Could you check a few things on this model? Use its own coordinates, in mm. Face numbers are marked on the shaded views. Round coordinates to 2 decimals unless told otherwise and drop trailing zeros. Loops run counter-clockwise (first coordinate to the right, second up) from the corner with the lowest first, then second, coordinate; pieces in that order, holes last. Notation, with made-up numbers: (84, 59.25) -> (92, 59.25) arc R36 ccw to (92, 95.25) -> close; hole circle Ø5 at (20, -17.5). An arc over 180 degrees is marked (long way). Write each question's results on one line, items separated by ' | '.
from build123d import *

# Parameters (mm, degrees)
SKETCH1_W           = 37.9349
SKETCH1_H           = 37.9349
BOSS_EXTRUDE1_DEPTH = 3.175
SKETCH9_R           = 1.1176
SKETCH9_R_2         = 6.35
CUT_EXTRUDE2_DEPTH  = 3.175


with BuildPart() as part:
    # Sketch1 → Boss-Extrude1 (new body)
    with BuildSketch(Plane.XY):
        with Locations((18.96745, 18.96745)):
            Rectangle(SKETCH1_W, SKETCH1_H)
    extrude(amount=BOSS_EXTRUDE1_DEPTH)

    # Sketch9 → Cut-Extrude2 (cut)
    with BuildSketch(Plane.XY.offset(3.175)):
        with Locations((33.62325, 33.62325)):
            Circle(SKETCH9_R)
        with Locations((4.31165, 33.62325)):
            Circle(SKETCH9_R)
        with Locations((4.31165, 4.31165)):
            Circle(SKETCH9_R)
        with Locations((33.62325, 4.31165)):
            Circle(SKETCH9_R)
        with Locations((18.96745, 18.96745)):
            Circle(SKETCH9_R_2)
        with BuildLine():
            Line((35.385619933, 12.100169933), (35.385619933, 2.549280067))
            Line((35.385619933, 2.549280067), (25.834730067, 2.549280067))
            ThreePointArc((25.834730067, 2.549280067), (25.2984, 2.01295), (25.834730067, 1.476619933))
            Line((25.834730067, 1.476619933), (35.385619933, 1.476619933))
            ThreePointArc((35.385619933, 1.476619933), (37.303202335, 0.631697665), (36.458280067, 2.549280067))
            Line((36.458280067, 2.549280067), (36.458280067, 12.100169933))
            ThreePointArc((36.458280067, 12.100169933), (35.92195, 12.6365), (35.385619933, 12.100169933))
        make_face()
        with BuildLine():
            Line((35.385619933, 36.458280067), (25.834730067, 36.458280067))
            ThreePointArc((25.834730067, 36.458280067), (25.2984, 35.92195), (25.834730067, 35.385619933))
            Line((25.834730067, 35.385619933), (35.385619933, 35.385619933))
            Line((35.385619933, 35.385619933), (35.385619933, 25.834730067))
            ThreePointArc((35.385619933, 25.834730067), (35.92195, 25.2984), (36.458280067, 25.834730067))
            Line((36.458280067, 25.834730067), (36.458280067, 35.385619933))
            ThreePointArc((36.458280067, 35.385619933), (37.303202335, 37.303202335), (35.385619933, 36.458280067))
        make_face()
        with BuildLine():
            Line((12.048880067, 36.458280067), (2.549280067, 36.458280067))
            ThreePointArc((2.549280067, 36.458280067), (0.631697665, 37.303202335), (1.476619933, 35.385619933))
            Line((1.476619933, 35.385619933), (1.476619933, 25.886019933))
            ThreePointArc((1.476619933, 25.886019933), (2.01295, 25.349689867), (2.549280067, 25.886019933))
            Line((2.549280067, 25.886019933), (2.549280067, 35.385619933))
            Line((2.549280067, 35.385619933), (12.048880067, 35.385619933))
            ThreePointArc((12.048880067, 35.385619933), (12.585210133, 35.92195), (12.048880067, 36.458280067))
        make_face()
        with BuildLine():
            Line((23.06955, 36.458280067), (14.86535, 36.458280067))
            ThreePointArc((14.86535, 36.458280067), (14.329019933, 35.92195), (14.86535, 35.385619933))
            Line((14.86535, 35.385619933), (23.06955, 35.385619933))
            ThreePointArc((23.06955, 35.385619933), (23.605880067, 35.92195), (23.06955, 36.458280067))
        make_face()
        with BuildLine():
            Line((2.549280067, 23.06955), (2.549280067, 14.86535))
            ThreePointArc((2.549280067, 14.86535), (2.01295, 14.329019933), (1.476619933, 14.86535))
            Line((1.476619933, 14.86535), (1.476619933, 23.06955))
            ThreePointArc((1.476619933, 23.06955), (2.01295, 23.605880067), (2.549280067, 23.06955))
        make_face()
        with BuildLine():
            Line((36.458280067, 23.06955), (36.458280067, 14.86535))
            ThreePointArc((36.458280067, 14.86535), (35.92195, 14.329019933), (35.385619933, 14.86535))
            Line((35.385619933, 14.86535), (35.385619933, 23.06955))
            ThreePointArc((35.385619933, 23.06955), (35.92195, 23.605880067), (36.458280067, 23.06955))
        make_face()
        with BuildLine():
            Line((23.06955, 2.549280067), (14.86535, 2.549280067))
            ThreePointArc((14.86535, 2.549280067), (14.329019933, 2.01295), (14.86535, 1.476619933))
            Line((14.86535, 1.476619933), (23.06955, 1.476619933))
            ThreePointArc((23.06955, 1.476619933), (23.605880067, 2.01295), (23.06955, 2.549280067))
        make_face()
        with BuildLine():
            Line((2.549280067, 12.100169933), (2.549280067, 2.549280067))
            Line((2.549280067, 2.549280067), (12.100169933, 2.549280067))
            ThreePointArc((12.100169933, 2.549280067), (12.6365, 2.01295), (12.100169933, 1.476619933))
            Line((12.100169933, 1.476619933), (2.600569933, 1.476619933))
            ThreePointArc((2.600569933, 1.476619933), (0.681867267, 0.681867267), (1.476619933, 2.600569933))
            Line((1.476619933, 2.600569933), (1.476619933, 12.100169933))
            ThreePointArc((1.476619933, 12.100169933), (2.01295, 12.6365), (2.549280067, 12.100169933))
        make_face()
    extrude(amount=-CUT_EXTRUDE2_DEPTH, mode=Mode.SUBTRACT)


solid = part.part
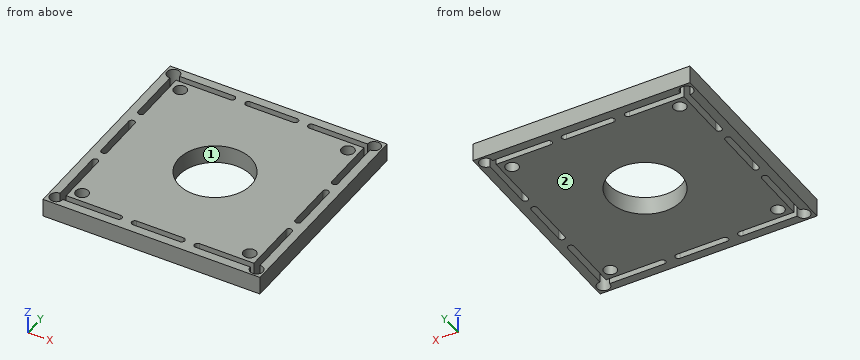
1) I'm going to push a flat-ended pin straight in: pin 1 (11.5 mm diameter, centred on x = 18.97, y = 18.97, fed in from +Z). Where does the tip first touch, or does it pass through?
Model answer:
pin 1: passes through
2) I want a section at A-A, the plane x = 27.5. Write out the boundary of the cut face in (y, z) (3 decimals), plus the area to 3 significant figures.
Model answer:
outline: (0, 0) -> (1.477, 0) -> (1.477, 3.175) -> (0, 3.175) -> close; (2.549, 0) -> (35.386, 0) -> (35.386, 3.175) -> (2.549, 3.175) -> close; (36.458, 0) -> (37.935, 0) -> (37.935, 3.175) -> (36.458, 3.175) -> close | area: 114 mm2
3) If we mould it in two halves opening along X, with no side actions, what happens to the marked faces 1 and 2? For each: released by +X, released by -X, zero draft, split by the parting line, or undercut.
Model answer:
face 1: undercut | face 2: zero draft
4) I need wall thicknesses on line 1 (X direction, y = 8, z = 2.9); line 2 (X direction, y = 33.5, z = 1.75). Which ranges of each line are inside material? Lowest first, please.
Model answer:
line 1: x = 0 to 1.48, 2.55 to 35.39, 36.46 to 37.93 | line 2: x = 0 to 1.48, 2.55 to 3.2, 5.42 to 32.51, 34.73 to 35.39, 36.46 to 37.93
5) I want a section at C-C, the plane y = 22.5. Write out the boundary of the cut face in (x, z) (3 decimals), plus the area to 3 significant figures.
Model answer:
outline: (0, 0) -> (1.477, 0) -> (1.477, 3.175) -> (0, 3.175) -> close; (2.549, 0) -> (13.691, 0) -> (13.691, 3.175) -> (2.549, 3.175) -> close; (24.244, 0) -> (35.386, 0) -> (35.386, 3.175) -> (24.244, 3.175) -> close; (36.458, 0) -> (37.935, 0) -> (37.935, 3.175) -> (36.458, 3.175) -> close | area: 80.1 mm2
6) I want a section at D-D, the plane z = 1.4. Give the number of separate pieces and of enclosed holes in the cut face, plus the area to 3 significant figures.
Model answer:
separate pieces: 1 | enclosed holes: 13 | area: 1,160 mm2
